Check sheet for the modelled part. Datum: model origin and axes. Units: mm. A direction names the side the tool comes from. Round coordinates to 2 decimals unless told otherwise and drop trailing zeros. Loops run counter-clockwise (first coordinate to the right, second up) from the corner with the lowest first, then second, coordinate; pieces in that order, holes last. Notation, with made-up numbers: (23.5, 82.25) -> (82.5, 82.25) arc R9 cw to (82.5, 93.25) -> close; hole circle Ø10 at (-25.75, -2.75). An arc over 180 degrees is marked (long way). Return JSON: item names as keys, results as strings.
from build123d import *

# Parameters (mm, degrees)
F1_DEPTH       = 35
F3_D           = 5
F3_START       = 1.7550021
F3_CBORE_D     = 10
F3_CBORE_DEPTH = 8
F4_W           = 22.4
F4_H           = 2
F5_DEPTH       = 25


with BuildPart() as f1:
    # F0 (on Top) → F1 (new body, symmetric)
    with BuildSketch(Plane.XY):
        with BuildLine():
            ThreePointArc((-17.0129362545, 4.1), (17.5, 0), (-17.0129362545, -4.1))
            Line((-17.0129362545, -4.1), (-27.8129362545, -4.1))
            Line((-27.8129362545, -4.1), (-27.8129362545, -12.5))
            ThreePointArc((-27.8129362545, -12.5), (-25.469790504, -18.1568542495), (-19.8129362545, -20.5))
            Line((-19.8129362545, -20.5), (0, -20.5))
            ThreePointArc((0, -20.5), (20.5, 0), (0, 20.5))
            Line((0, 20.5), (-19.8129362545, 20.5))
            ThreePointArc((-19.8129362545, 20.5), (-25.469790504, 18.1568542495), (-27.8129362545, 12.5))
            Line((-27.8129362545, 12.5), (-27.8129362545, 4.1))
            Line((-27.8129362545, 4.1), (-17.0129362545, 4.1))
        make_face()
    extrude(amount=F1_DEPTH, both=True)

    # F3 (through all)
    # its depths count from where the whole tool has entered the part; down to there all is cleared
    with Locations(Plane(origin=(0, 20.5, 0), x_dir=(-1, 0, 0), z_dir=(0, 1, 0)).offset(-F3_START)):
        with Locations((19.8129362545, -24.25), (19.8129362545, -9.25), (19.8129362545, 9.25), (19.8129362545, 24.25)):
            CounterBoreHole(F3_D / 2, F3_CBORE_D / 2, F3_CBORE_DEPTH)

    # F4 (on Front) → F5 (cut)
    with BuildSketch(Plane.XZ):
        with Locations((-16.6129362545, 0)):
            Rectangle(F4_W, F4_H)
    extrude(amount=-F5_DEPTH, mode=Mode.SUBTRACT)


solid = f1.part
Q1. Draft check along Y on faces 1 (the cylindrical face through (-21.8, 7.38, 7.73)), 2 (the flat face through (-5, 20.5, 0)), 3 (the flat face through (-22, 4.1, 18)). Enter one of: released by +Y, released by -Y, zero draft, split by the parting line, or undercut.
Results list:
{"face 1": "zero draft", "face 2": "released by +Y", "face 3": "undercut"}
Q2. Section check D-D (y = 15.5). Record the boundary of the cut face in (x, z).
Results list:
{"outline": "(-27.23, -35) -> (-8.12, -35) -> (-8.12, -1) -> (-27.23, -1) -> close; (-27.23, 1) -> (-8.12, 1) -> (-8.12, 35) -> (-27.23, 35) -> close; (8.12, -35) -> (13.42, -35) -> (13.42, 35) -> (8.12, 35) -> close; hole circle Ø10 at (-19.81, -24.25); hole circle Ø10 at (-19.81, -9.25); hole circle Ø10 at (-19.81, 9.25); hole circle Ø10 at (-19.81, 24.25)"}
Q3. Section check B-B (x = -10.5). Record the boundary of the cut face in (y, z), then the cut area to 3 significant figures.
Results list:
{"outline": "(-20.5, -35) -> (-14, -35) -> (-14, 35) -> (-20.5, 35) -> close; (14, -35) -> (20.5, -35) -> (20.5, -1) -> (14, -1) -> close; (14, 1) -> (20.5, 1) -> (20.5, 35) -> (14, 35) -> close", "area": "897 mm^2"}
Q4. Material ranges on line 1 (Y direction, x = -20, z = -29) (3 decimals); line 2 (X direction, y = 14, z = -12.5); line 3 (Y direction, x = 0, z = -5), recorded low to high.
Results list:
{"line 1": "-20.498 to -4.1, 4.1 to 10.745", "line 2": "-27.67 to -23.61, -16.01 to -10.5, 10.5 to 14.97", "line 3": "-20.5 to -17.5, 17.5 to 20.5"}
Q5. Section check A-A (y = -11.5). Record the boundary of the cut face in (x, z), then the cut area to 3 significant figures.
Results list:
{"outline": "(-27.81, -35) -> (-13.19, -35) -> (-13.19, 35) -> (-27.81, 35) -> close; (13.19, -35) -> (16.97, -35) -> (16.97, 35) -> (13.19, 35) -> close; hole circle Ø5 at (-19.81, -24.25); hole circle Ø5 at (-19.81, -9.25); hole circle Ø5 at (-19.81, 9.25); hole circle Ø5 at (-19.81, 24.25)", "area": "1,210 mm^2"}
Q6. Go/stop test with flat-tipped pins: pin 1 (12 mm diameter, centred on x = -22.5, z = -9.5, fed in from +Y); pin 2 (12 mm diameter, centred on y = 11, z = 8.5, fed in from +X); pin 3 (1.5 mm diameter, centred on x = -21.5, z = 10.5, fed in from -Y); pin 4 (3 mm diameter, centred on x = -18, z = 10, fed in from +Y) (3 decimals). Record where each tip stops, or that it passes through.
Results list:
{"pin 1": "y = 20.5", "pin 2": "x = 19.88", "pin 3": "y = -20.35", "pin 4": "y = 10.745"}
Q7. Section check C-C (z = 24.25). Record the boundary of the cut face in (x, y) (3 decimals), then the cut area to 3 significant figures.
Results list:
{"outline": "(-27.813, -12.5) arc R8 ccw to (-22.313, -20.099) -> (-22.313, -4.1) -> (-27.813, -4.1) -> close; (-27.813, 4.1) -> (-22.313, 4.1) -> (-22.313, 10.745) -> (-24.813, 10.745) -> (-24.813, 18.745) arc R8 ccw to (-27.813, 12.5) -> close; (-17.313, -20.5) -> (0, -20.5) arc R20.5 ccw to (0, 20.5) -> (-14.813, 20.5) -> (-14.813, 10.745) -> (-17.313, 10.745) -> (-17.313, 4.1) -> (-17.013, 4.1) arc R17.5 cw (long way) to (-17.013, -4.1) -> (-17.313, -4.1) -> close", "area": "515 mm^2"}
Q8. Tool access check on faces 4 (the cylindrical face through (-21.656, -12.415, 25.94)), 5 (the flat face through (-22, 4.1, -18)), 6 (the cylindrical face through (-14.818, 15.691, -24.03)). Record the directions out of +Z, -Z, +X, -X, +Y, -Y that give a thin tool (end or side, any length) a straight path to the whole face; none if there is none.
Results list:
{"face 4": "+Y, -Y", "face 5": "+Z, -Z, -X", "face 6": "+Y"}
